Can you work these out from the model? Positions are in its coordinate system, mm. A direction names the side the tool comes from. Coordinates: 2 decimals unless noted, no trailing zeros. Order: outer loops, then holes, each group sorted by start corner. A loop starts at its lowest first (then second) coordinate and runs counter-clockwise, first axis right, second up. Notation, with made-up numbers: (-11, 29.5) - (3, 29.5) arc R5 ccw to (3, 35.5) - close; hole circle Ø2 at (-6, 20). An arc over 180 degrees is marked (long way). Use a Markdown table: item, result. Add a question column.
(1) I want a section at B-B (z = -9). List the corners of the cut face in (x, y) for me, and give its area (3 significant figures).
(2) If I drill on L1, parallel to Z at x = -11.45, y = 3.5; L2, parallel to Z at x = -12.65, y = 2.25; L3, parallel to X at y = 5.5, z = 6.5, over which ranges is the centre line in solid material (lowest first)? Write a range as [from, to].
(3) For pin 1 Ø0.6 at (x, z) = (-12, 12.5) entering from -Y; pin 2 Ø7.5 at (y, z) = (-5, -17) entering from -X; pin 3 Ø5.5 at (y, z) = (13, 13) entering from +X, each with a flat end and sliding along its axis, tell me the tip position at first contact or that it passes through.
(4) On a 3-axis mill with a long thin cutter (end or side, diameter ignored), from which of +Z, -Z, +X, -X, +Y, -Y can I reach the whole of each face in a straight line? I mean faces 4 (the flat face through (-12, 7, -18.044)), 5 (the flat face through (-11.016, 13, 10)), 6 (the flat face through (-12, 7, 10)). Say none if no direction works.
(5) We'd pull the mould along X, two halves only. Please class faces 1 (the flat face through (-13, 0, -3)), 2 (the flat face through (-14.296, 5, -3)), 3 (the flat face through (-12, 3, 22.942)): pulls with the +X half, pulls with the -X half, needs draft (parallel to the pull), parting line crosses it, or undercut.
(6) I want a section at A-A (x = -11.8). List the corners of the cut face in (y, z) for me.
(7) I want a section at D-D (z = -19.5). List the corners of the cut face in (x, y) for me, and give its area (3 significant figures).
(8) I want a section at C-C (y = -5). List the corners of the cut face in (x, z) for me, and give its area (3 significant figures).
```python
from build123d import *

# Parameters (mm, degrees)
SKETCH1_W           = 4.980670257
SKETCH1_H           = 54.9718421
BOSS_EXTRUDE1_DEPTH = 10
SKETCH2_W           = 1.980670257
SKETCH2_H           = 15
CUT_EXTRUDE2_DEPTH  = 7
SKETCH4_W           = 1.980670257
SKETCH4_H           = 25.98592105
CUT_EXTRUDE3_DEPTH  = 7
SKETCH5_W           = 1.580670257
SKETCH5_H           = 25.78592105
BOSS_EXTRUDE2_DEPTH = 7
SKETCH6_W           = 1.580670257
SKETCH6_H           = 25.78592105
BOSS_EXTRUDE3_DEPTH = 7


with BuildPart() as part:
    # Sketch1 → Boss-Extrude1 (new body)
    with BuildSketch(Plane(origin=(0, 0, 0), x_dir=(1, 0, 0), z_dir=(0, 1, 0))):
        with Locations((-11.806033203, 3.043742935)):
            Rectangle(SKETCH1_W, SKETCH1_H)
    extrude(amount=BOSS_EXTRUDE1_DEPTH)

    # Sketch2 → Cut-Extrude2 (cut)
    with BuildSketch(Plane(origin=(0, 10, 0), x_dir=(1, 0, 0), z_dir=(0, 1, 0))):
        with Locations((-11.806033203, 10.543742935)):
            Rectangle(SKETCH2_W, SKETCH2_H)
    extrude(amount=-CUT_EXTRUDE2_DEPTH, mode=Mode.SUBTRACT)

    # Sketch4 → Cut-Extrude3 (cut)
    with BuildSketch(Plane.XZ):
        with Locations((-11.806033203, 9.94921759)):
            Rectangle(SKETCH4_W, SKETCH4_H)
    extrude(amount=-CUT_EXTRUDE3_DEPTH, mode=Mode.SUBTRACT)

    # Sketch5 → Boss-Extrude2 (add)
    with BuildSketch(Plane.XZ):
        with Locations((-11.806033203, -15.93670346)):
            Rectangle(SKETCH5_W, SKETCH5_H)
    extrude(amount=BOSS_EXTRUDE2_DEPTH)

    # Sketch6 → Boss-Extrude3 (add)
    with BuildSketch(Plane(origin=(0, 10, 0), x_dir=(1, 0, 0), z_dir=(0, 1, 0))):
        with Locations((-11.806033203, -9.84921759)):
            Rectangle(SKETCH6_W, SKETCH6_H)
    extrude(amount=BOSS_EXTRUDE3_DEPTH)


solid = part.part
```
Answers follow:
| question | item | result |
|---|---|---|
| 1 | outline | (-14.3, 0) - (-12.6, 0) - (-12.6, -7) - (-11.02, -7) - (-11.02, 0) - (-9.32, 0) - (-9.32, 10) - (-10.82, 10) - (-10.82, 3) - (-12.8, 3) - (-12.8, 10) - (-14.3, 10) - close |
| 1 | area | 47.0 mm² |
| 2 | L1 | z = [-30.53, -18.04], [22.94, 24.44] |
| 2 | L2 | z = [-30.53, -3.04], [22.94, 24.44] |
| 2 | L3 | x = [-14.3, -12.8], [-10.82, -9.32] |
| 3 | pin 1 | stops at y = 7 |
| 3 | pin 2 | stops at x = -12.6 |
| 3 | pin 3 | stops at x = -11.02 |
| 4 | face 4 | +Y |
| 4 | face 5 | +Z, -Z, +X, +Y |
| 4 | face 6 | -Y |
| 5 | face 1 | needs draft |
| 5 | face 2 | pulls with the -X half |
| 5 | face 3 | undercut |
| 6 | outline | (-7, -28.83) - (0, -28.83) - (0, -30.53) - (10, -30.53) - (10, -18.04) - (3, -18.04) - (3, -3.04) - (-7, -3.04) - close; (0, 22.94) - (7, 22.94) - (7, -3.04) - (17, -3.04) - (17, 22.74) - (10, 22.74) - (10, 24.44) - (0, 24.44) - close |
| 7 | outline | (-14.3, 0) - (-12.6, 0) - (-12.6, -7) - (-11.02, -7) - (-11.02, 0) - (-9.32, 0) - (-9.32, 10) - (-14.3, 10) - close |
| 7 | area | 60.9 mm² |
| 8 | outline | (-12.6, -28.83) - (-11.02, -28.83) - (-11.02, -3.04) - (-12.6, -3.04) - close |
| 8 | area | 40.8 mm² |
